Here's how the part is built. I have some questions about the finished solid (model axes, mm). A direction names the side the tool comes from. Give positions to 0.01 mm unless a question says otherwise; leave off trailing zeros. Loops run counter-clockwise (first coordinate to the right, second up) from the corner with the lowest first, then second, coordinate; pieces in that order, holes last. Notation, with made-up numbers: (35, -25.5) - (72, -25.5) arc R20 cw to (72, -2.5) - close; hole circle Ø9 at (86, -8). An arc over 180 degrees is marked (long way). Put each result on its own line as item: value. Start each with the question number.
from build123d import *

# Parameters (mm, degrees)
SKETCH1_R           = 3.5
BOSS_EXTRUDE2_DEPTH = 55
SKETCH7_W           = 68.999652055
SKETCH7_H           = 50.415620377
CUT_EXTRUDE5_DEPTH  = 13
SKETCH19_W          = 74.859412742
SKETCH19_H          = 60.725118028
CUT_EXTRUDE7_DEPTH  = 13


with BuildPart() as part:
    # Sketch1 → Boss-Extrude2 (new body)
    with BuildSketch(Plane(origin=(0, 0, 0), x_dir=(1, 0, 0), z_dir=(0, 1, 0))):
        with BuildLine():
            Line((-77.08996548, -66.932643829), (112.637979465, -57.343127962))
            add(Edge.make_bspline(
                [(112.637979465, -57.343127962), (125.082628436, -56.027724614), (133.287763268, -44.662014668), (142.702606635, -37.943127962)],
                knots=[0, 0, 0, 0, 1, 1, 1, 1], degree=3))
            Line((142.702606635, -37.943127962), (146.202606635, -37.943127962))
            Line((146.202606635, -37.943127962), (146.302606635, -37.943127962))
            ThreePointArc((146.302606635, -37.943127962), (150.120983253, -36.36150458), (151.702606635, -32.543127962))
            Line((151.702606635, -32.543127962), (151.702606635, 23.656872038))
            ThreePointArc((151.702606635, 23.656872038), (150.120983253, 27.475248656), (146.302606635, 29.056872038))
            Line((146.302606635, 29.056872038), (146.202606635, 29.056872038))
            Line((146.202606635, 29.056872038), (142.702606635, 29.056872038))
            add(Edge.make_bspline(
                [(112.637979465, 48.456872038), (125.082628436, 47.14146869), (133.287763268, 35.775758744), (142.702606635, 29.056872038)],
                knots=[0, 0, 0, 0, 1, 1, 1, 1], degree=3))
            Line((112.637979465, 48.456872038), (-77.08996548, 58.046387905))
            add(Edge.make_bspline(
                [(-77.08996548, 58.046387905), (-97.502880255, 56.762508137), (-92.602876077, 31.29935649), (-112.297393365, 29.056872038)],
                knots=[0, 0, 0, 0, 1, 1, 1, 1], degree=3))
            Line((-112.297393365, 29.056872038), (-115.797393365, 29.056872038))
            Line((-115.797393365, 29.056872038), (-115.897393365, 29.056872038))
            ThreePointArc((-115.897393365, 29.056872038), (-119.715769983, 27.475248656), (-121.297393365, 23.656872038))
            Line((-121.297393365, 23.656872038), (-121.297393365, -32.543127962))
            ThreePointArc((-121.297393365, -32.543127962), (-119.715769983, -36.36150458), (-115.897393365, -37.943127962))
            Line((-115.897393365, -37.943127962), (-115.797393365, -37.943127962))
            Line((-115.797393365, -37.943127962), (-112.297393365, -37.943127962))
            add(Edge.make_bspline(
                [(-77.08996548, -66.932643829), (-97.502880255, -65.648764061), (-92.602876077, -40.185612414), (-112.297393365, -37.943127962)],
                knots=[0, 0, 0, 0, 1, 1, 1, 1], degree=3))
        make_face()
        with Locations((-112.297393365, 20.556872038)):
            Circle(SKETCH1_R, mode=Mode.SUBTRACT)
        with Locations((-112.297393365, -29.443127962)):
            Circle(SKETCH1_R, mode=Mode.SUBTRACT)
        with Locations((142.702606635, -29.443127962)):
            Circle(SKETCH1_R, mode=Mode.SUBTRACT)
        with Locations((142.702606635, 20.556872038)):
            Circle(SKETCH1_R, mode=Mode.SUBTRACT)
        with BuildLine():
            Line((-75.675939266, -60.937869235), (111.223953251, -52.297869235))
            add(Edge.make_bspline(
                [(111.223953251, -52.297869235), (116.613661153, -51.728175398), (121.119803585, -49.063877422), (125.288889488, -45.778967713)],
                knots=[0, 0, 0, 0, 0.481216011, 0.481216011, 0.481216011, 0.481216011], degree=3))
            Line((125.288889488, -45.778967713), (125.288889488, 36.892711789))
            add(Edge.make_bspline(
                [(111.223953251, 42.922130765), (116.613661153, 41.934143872), (121.119803585, 40.177621498), (125.288889488, 36.892711789)],
                knots=[0, 0, 0, 0, 0.481216011, 0.481216011, 0.481216011, 0.481216011], degree=3))
            Line((111.223953251, 42.922130765), (-75.675939266, 51.562130765))
            add(Edge.make_bspline(
                [(-75.675939266, 51.562130765), (-87.01186848, 49.517204736), (-89.586983119, 42.038204428), (-94.215939266, 34.771613311)],
                knots=[0, 0, 0, 0, 0.62412853, 0.62412853, 0.62412853, 0.62412853], degree=3))
            Line((-94.215939266, 34.771613311), (-94.215939266, -43.657869235))
            add(Edge.make_bspline(
                [(-75.675939266, -60.937869235), (-87.01186848, -60.09623443), (-89.586983119, -50.924460352), (-94.215939266, -43.657869235)],
                knots=[0, 0, 0, 0, 0.62412853, 0.62412853, 0.62412853, 0.62412853], degree=3))
        make_face(mode=Mode.SUBTRACT)
    extrude(amount=-BOSS_EXTRUDE2_DEPTH)

    # Sketch7 → Cut-Extrude5 (cut)
    with BuildSketch(Plane.ZY.offset(121.297393365)):
        with Locations((4.333112833, -30.707810189)):
            Rectangle(SKETCH7_W, SKETCH7_H)
    extrude(amount=-CUT_EXTRUDE5_DEPTH, mode=Mode.SUBTRACT)

    # Sketch19 → Cut-Extrude7 (cut)
    with BuildSketch(Plane(origin=(151.702606635, 0, 0), x_dir=(0, 0, -1), z_dir=(1, 0, 0))):
        with Locations((-5.097493458, -35.862559014)):
            Rectangle(SKETCH19_W, SKETCH19_H)
    extrude(amount=-CUT_EXTRUDE7_DEPTH, mode=Mode.SUBTRACT)


solid = part.part
1) Thinking about a two-plate mould opening in Z: for faces 4 (the flat face through (35, 0, -47)), 5 (the flat face through (19.102, -27.115, -53.185)), 6 (the flat face through (16.446, -27.115, 62.205)), 7 (the cylindrical face through (145.936, -2.712, 30.784)), which applies, pulls with the +Z half, pulls with the -Z half, needs draft (parallel to the pull), parting line crosses it, or undercut?
2) I need wall thicknesses on line 1 (X direction, y = -10, z = 24.5); line 2 (Z direction, x = -44.5, y = -10); line 3 (Z direction, x = -34, y = -18.5). Which ranges of each line are inside material? Lowest first, please.
3) Suppose I cut it at C-C on x = 38. Please give me the cut outline in (y, z), plus the area to 3 significant figures.
4) Suppose I cut it at B-B on x = 73.5. Please give me the cut outline in (y, z).
5) I'm going to push flat-ended pins straight in: P1, Ø8, axis at y = -18, z = 23.5, coming from the +X side; P2, Ø4, axis at x = 143, z = -9.5, coming from the -Y side; P3, Ø3, axis at x = 145, y = -4, coming from the -Z side; P4, Ø10.5, axis at x = -112, z = 5, coming from the -Y side. Where does each tip first touch, or does it pass through?
6) Suppose I cut it at A-A on z = -8. Please give me the cut outline in (x, y).
7) Which directions (+Z, -Z, +X, -X, +Y, -Y) give clear straight access to the entire face, cutting with the end or side of a thin tool? Please do faces 1 (the flat face through (138.703, -30, 5)), 2 (the flat face through (-115, -5.5, 4)), 3 (the flat face through (-94.216, -27, 4)).
Ans:
1. face 4: needs draft
1. face 5: pulls with the -Z half
1. face 6: pulls with the +Z half
1. face 7: undercut
2. line 1: x = -108.3 to -94.22, 125.29 to 138.7
2. line 2: z = -56.4 to -50.12, 59.5 to 65.29
2. line 3: z = -55.87 to -49.64, 59.01 to 64.75
3. outline: (-55, -52.23) - (0, -52.23) - (0, -46.31) - (-55, -46.31) - close; (-55, 55.68) - (0, 55.68) - (0, 61.12) - (-55, 61.12) - close
3. area: 625 mm²
4. outline: (-55, -50.44) - (0, -50.44) - (0, -44.67) - (-55, -44.67) - close; (-55, 54.04) - (0, 54.04) - (0, 59.32) - (-55, 59.32) - close
5. P1: stops at x = 138.7
5. P2: stops at y = -5.5
5. P3: stops at z = -29.06
5. P4: stops at y = -55
6. outline: (-121.3, -5.5) - (-108.3, -5.5) - (-108.3, -55) - (-94.22, -55) - (-94.22, 0) - (-121.3, 0) - close; (125.29, -55) - (138.7, -55) - (138.7, -5.5) - (151.7, -5.5) - (151.7, 0) - (125.29, 0) - close
7. face 1: +Z, -Z, +X, -Y
7. face 2: +Z, -Z, -X, -Y
7. face 3: +Y, -Y
